from build123d import *

# Parameters (mm, degrees)
SKETCH2_R           = 4.5
BOSS_EXTRUDE1_DEPTH = 92


with BuildPart() as part:
    # Sketch1 → Revolve1 (revolve)
    with BuildSketch(Plane(origin=(0, 0, 0), x_dir=(0, 0, -1), z_dir=(1, 0, 0))):
        Polygon((0, 0), (34.5, 0), (34.5, -2), (31, -2), (31, -6), (34.5, -6), (34.5, -14), (34.5, -18), (34.5, -20), (0, -20), align=None)
    revolve(axis=Axis((0, -20, 0), (0, 1, 0)))

    # Sketch2 → Boss-Extrude1 (add)
    with BuildSketch(Plane.XZ.offset(20)):
        Circle(SKETCH2_R)
    extrude(amount=BOSS_EXTRUDE1_DEPTH)


solid = part.part
Geometry: final body of the model. Coordinates: model frame, mm. A direction names the side the tool comes from. Give positions to 0.01 mm unless a question says otherwise; leave off trailing zeros. Write each loop counter-clockwise with the first axis right and the second up, starting at its lowest first coordinate (ties: lowest second). Pieces come first, ordered by that corner, then holes.
(1) Access query for faces 1 (the flat face through (-18, -2, 26)), 2 (the cylindrical face through (-10.363, -12.902, -32.907)). Directions: +Z, -Z, +X, -X, +Y, -Y. A direction counts if a zero-diameter tool reaches every point of the face in a straight line with its end or side. Return the directions, or none.
(2) Cut plane A-A, the plane x = 0. Return loops of the section in (y, z), then the cut area to 3 significant figures.
(3) Cut plane B-B, the plane z = 0. Return loops of the section in (x, y).
(4) Mould query, pull axis Y, two halves, no side actions, for faces 3 (the cylindrical face through (-30.736, -4.028, 4.036)), 4 (the flat face through (-18, -6, -26)), 5 (the cylindrical face through (-0.59, -65.36, 4.46)), 6 (the flat face through (0, 0, 0)). Classes: released by +Y, released by -Y, zero draft, split by the parting line, or undercut.
(5) Cut plane D-D, the plane z = 11.5. Return loops of the section in (x, y).
(6) Ray query, line 1 (Y direction, x = -21, z = 26.5); line 2 (Y direction, x = -24, z = -10); line 3 (Z direction, x = 3, y = -41.5). Return the intervals inside material, ascending.
(7) First-contact query: P1, Ø10, axis at x = 24, z = 3.5, coming from the -Y side; P2, Ø5, axis at y = -14.5, z = 20.5, coming from the +X side. Flat tips, straight axial feed; report the tip coordinate or a pass-through.
(8) Cut plane C-C, the plane y = -41. Return loops of the section in (x, z), then the cut area to 3 significant figures.
Values follow:
1. face 1: none
1. face 2: +Y, -Y
2. outline: (-112, -4.5) - (-20, -4.5) - (-20, -34.5) - (-6, -34.5) - (-6, -31) - (-2, -31) - (-2, -34.5) - (0, -34.5) - (0, 34.5) - (-2, 34.5) - (-2, 31) - (-6, 31) - (-6, 34.5) - (-20, 34.5) - (-20, 4.5) - (-112, 4.5) - close
2. area: 2,180 mm2
3. outline: (-34.5, -20) - (-4.5, -20) - (-4.5, -112) - (4.5, -112) - (4.5, -20) - (34.5, -20) - (34.5, -6) - (31, -6) - (31, -2) - (34.5, -2) - (34.5, 0) - (-34.5, 0) - (-34.5, -2) - (-31, -2) - (-31, -6) - (-34.5, -6) - close
4. face 3: undercut
4. face 4: undercut
4. face 5: zero draft
4. face 6: released by +Y
5. outline: (-32.53, -20) - (32.53, -20) - (32.53, -6) - (28.79, -6) - (28.79, -2) - (32.53, -2) - (32.53, 0) - (-32.53, 0) - (-32.53, -2) - (-28.79, -2) - (-28.79, -6) - (-32.53, -6) - close
6. line 1: y = -20 to -6, -2 to 0
6. line 2: y = -20 to 0
6. line 3: z = -3.35 to 3.35
7. P1: stops at y = -20
7. P2: stops at x = 29.43
8. outline: circle Ø9 at (0, 0)
8. area: 63.6 mm2
